Input: part model. Units: mm. Frame: model coordinates. Give positions to 0.01 mm unless a question says otherwise; leave off trailing zeros. Order: outer loops, then holes, each group sorted by start corner. A loop starts at its lowest first (then second) coordinate and runs counter-clockwise, first axis right, second up. Notation, with made-up numbers: (-10.5, 49.25) - (-1.5, 49.25) arc R11 ccw to (-1.5, 67.25) - close; hole circle Ø11 at (44.5, -40). An arc over 180 degrees is marked (long way). Use a Markdown table: item, result.
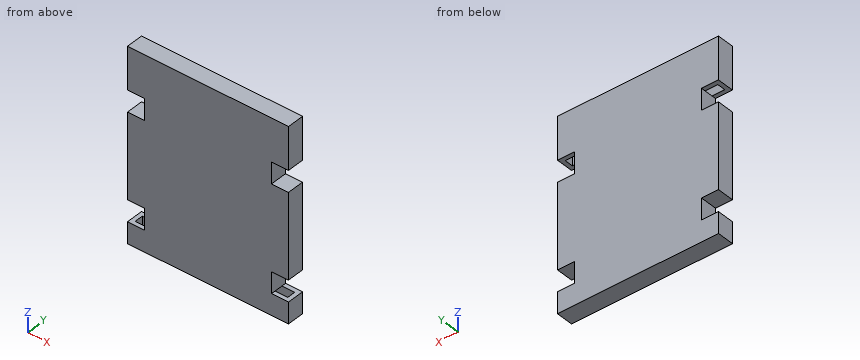
from build123d import *

# Parameters (mm, degrees)
F0_W     = 10.16
F0_H     = 12.7
F0_H_2   = 50.8
F0_H_3   = 25.4
F1_DEPTH = 5.08
F2_T     = -2.54


# Not quite as in the source:
# - a shell that OpenCascade refuses in one call is made with other operations: the cavity is built on its own and cut out


with BuildPart() as f1:
    # F0 (on Front) → F1 (new body, symmetric)
    with BuildSketch(Plane.XZ):
        Polygon((-38.1, -57.15), (38.1, -57.15), (38.1, -44.45), (38.1, -31.75), (38.1, 19.05), (38.1, 31.75), (38.1, 57.15), (-38.1, 57.15), (-38.1, 31.75), (-38.1, 19.05), (-38.1, -31.75), (-38.1, -44.45), align=None)
        with Locations((43.18, -50.8)):
            Rectangle(F0_W, F0_H)
        with Locations((-43.18, -50.8)):
            Rectangle(F0_W, F0_H)
        with Locations((43.18, -6.35)):
            Rectangle(F0_W, F0_H_2)
        with Locations((-43.18, -6.35)):
            Rectangle(F0_W, F0_H_2)
        with Locations((43.18, 44.45)):
            Rectangle(F0_W, F0_H_3)
        with Locations((-43.18, 44.45)):
            Rectangle(F0_W, F0_H_3)
    extrude(amount=F1_DEPTH, both=True)

    # F2: a shell. OpenCascade refuses it in one call, so the cavity is built on its own and cut out:
    # the body offset inwards by the wall thickness, plus a prism from it out through each open face.
    f2_core = offset(f1.part, amount=F2_T, kind=Kind.INTERSECTION, mode=Mode.PRIVATE)
    f2_exits = [f2_core.faces().sort_by_distance(p)[0] for p in [
        (40.64, 0, 34.29),
        (40.64, 0, -46.99),
        (-40.64, 0, -46.99),
        (-40.64, 0, 34.29),
    ]]
    add(f2_core, mode=Mode.SUBTRACT)
    extrude(f2_exits, amount=-F2_T, mode=Mode.SUBTRACT)


solid = f1.part
1. Section query C-C (x = -27). Return loops of the section in (y, z), then the cut area to 3 significant figures.
Response:
| item | result |
|---|---|
| outline | (-5.08, -57.15) - (5.08, -57.15) - (5.08, 57.15) - (-5.08, 57.15) - close; hole (-2.54, -54.61) - (2.54, -54.61) - (2.54, 54.61) - (-2.54, 54.61) - close |
| area | 606 mm^2 |
2. Section query B-B (z = 21). Return loops of the section in (x, y).
Response:
| item | result |
|---|---|
| outline | (-38.1, -5.08) - (38.1, -5.08) - (38.1, 5.08) - (-38.1, 5.08) - close; hole (-35.56, -2.54) - (35.56, -2.54) - (35.56, 2.54) - (-35.56, 2.54) - close |
3. Section query A-A (x = 42). Return loops of the section in (y, z).
Response:
| item | result |
|---|---|
| outline | (-5.08, -57.15) - (5.08, -57.15) - (5.08, -44.45) - (2.54, -44.45) - (2.54, -54.61) - (-2.54, -54.61) - (-2.54, -44.45) - (-5.08, -44.45) - close; (-5.08, -31.75) - (5.08, -31.75) - (5.08, 19.05) - (-5.08, 19.05) - close; (-5.08, 31.75) - (-2.54, 31.75) - (-2.54, 54.61) - (2.54, 54.61) - (2.54, 31.75) - (5.08, 31.75) - (5.08, 57.15) - (-5.08, 57.15) - close; hole (-2.54, -29.21) - (2.54, -29.21) - (2.54, 16.51) - (-2.54, 16.51) - close |
4. Material intervals for line 1 along Z through (x, y) = (-38, 2.5); line 2 along Z through (x, y) = (-39, -0.25); line 3 along Y through (x, z) = (14.5, -7.5), sorted ascending.
Response:
| item | result |
|---|---|
| line 1 | z = -57.15 to -54.61, -44.45 to -29.21, 16.51 to 31.75, 54.61 to 57.15 |
| line 2 | z = -57.15 to -54.61, -31.75 to -29.21, 16.51 to 19.05, 54.61 to 57.15 |
| line 3 | y = -5.08 to -2.54, 2.54 to 5.08 |
5. Section query D-D (y = 0.75). State how many separate pieces and enclosed holes the cut face has, then the cut area to 3 significant figures.
Response:
| item | result |
|---|---|
| separate pieces | 4 |
| enclosed holes | 0 |
| area | 1,150 mm^2 |
6. Pin query (flat end, axial travel): pin 1 (3 mm diameter, centred on y = 0.5, z = 24, fed in from -X); pin 2 (5.5 mm diameter, centred on y = 0.5, z = -36, fed in from +X). Return the tip coordinate at first contact, or that it passes through.
Response:
| item | result |
|---|---|
| pin 1 | stops at x = -38.1 |
| pin 2 | stops at x = 38.1 |
